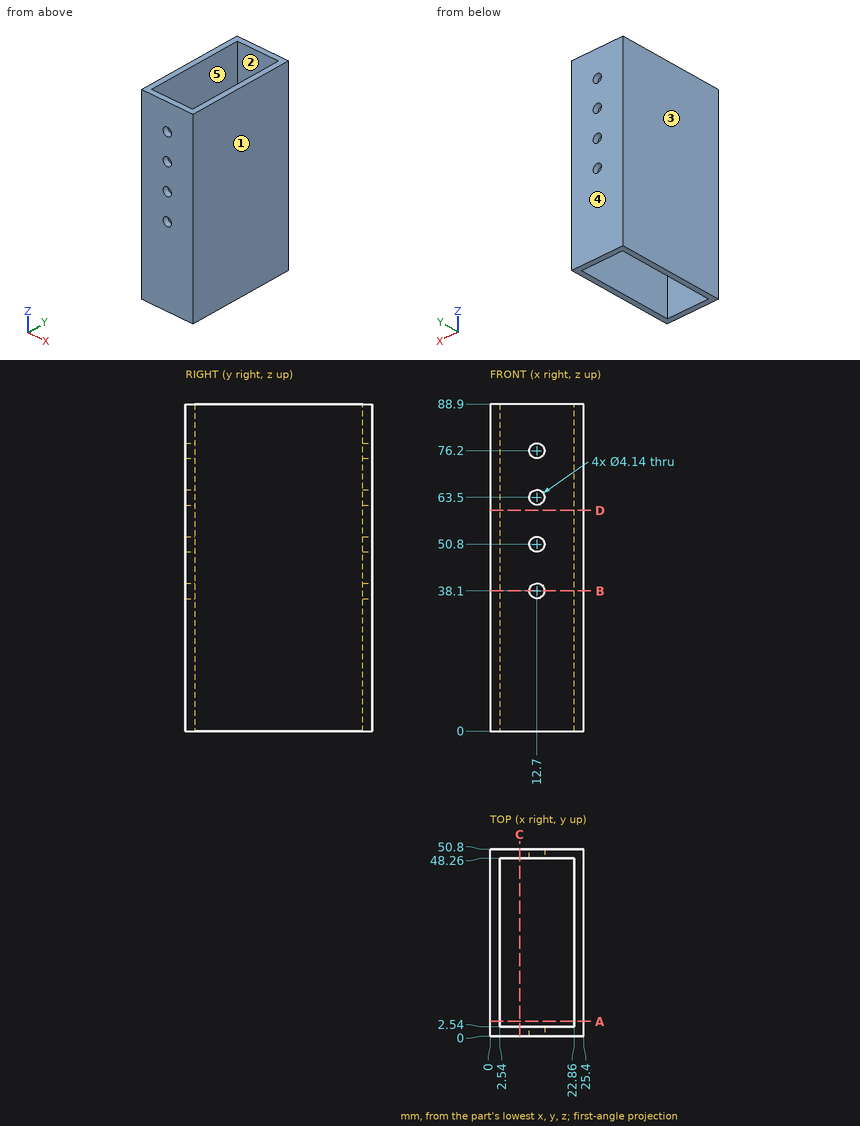
Answer from the drawing. Dimensions are ordinates in mm from the lowest x, y and z of the part. A direction names the side the tool comes from. Round coordinates to 2 decimals unless told otherwise and drop trailing zeros. Loops run counter-clockwise (first coordinate to the right, second up) from the corner with the lowest first, then second, coordinate; pieces in that order, holes last.
Q1. This flat-tipped pin is pushed along its axis until it touches: pin 1 (2.5 mm diameter, centred on x = 12.7, z = 38.1, fed in from +Y). Where does it stop, or does it pass through?
Q2. Determine the mould class of the marked faces 3, 4 and 5 for opening direction Y: released by +Y, released by -Y, zero draft, split by the parting line, or undercut.
Q3. Section D-D on z = 60 is taken. Write down the section's boundary in (x, y), and give its area (3 significant figures).
Q4. Section A-A on y = 4 is taken. Write down the section's boundary in (x, z).
Q5. Section B-B on z = 38.1 is taken. Write down the section's boundary in (x, y).
Q6. Consider probe 1 along Z at (x, y) = (12.7, 0.6); probe 2 along X at (y, z) = (37.5, 16.5); probe 3 along Y at (x, z) = (15.5, 12.5). Determine where each line is inside the solid, lowest interval first.
Q7. Which of the six approach directions +Z, -Z, +X, -X, +Y, -Y give full straight-line access (tool end or side, diameter ignored) to the marked faces 1 and 2?
Q8. Section C-C on x = 8 is taken. Write down the section's boundary in (y, z).
Output:
1. pin 1: passes through
2. face 3: zero draft
2. face 4: released by +Y
2. face 5: undercut
3. outline: (0, 0) - (25.4, 0) - (25.4, 50.8) - (0, 50.8) - close; hole (2.54, 2.54) - (22.86, 2.54) - (22.86, 48.26) - (2.54, 48.26) - close
3. area: 361 mm2
4. outline: (0, 0) - (2.54, 0) - (2.54, 88.9) - (0, 88.9) - close; (22.86, 0) - (25.4, 0) - (25.4, 88.9) - (22.86, 88.9) - close
5. outline: (0, 0) - (10.63, 0) - (10.63, 2.54) - (2.54, 2.54) - (2.54, 48.26) - (10.63, 48.26) - (10.63, 50.8) - (0, 50.8) - close; (14.77, 0) - (25.4, 0) - (25.4, 50.8) - (14.77, 50.8) - (14.77, 48.26) - (22.86, 48.26) - (22.86, 2.54) - (14.77, 2.54) - close
6. probe 1: z = 0 to 36.03, 40.17 to 48.73, 52.87 to 61.43, 65.57 to 74.13, 78.27 to 88.9
6. probe 2: x = 0 to 2.54, 22.86 to 25.4
6. probe 3: y = 0 to 2.54, 48.26 to 50.8
7. face 1: +Z, -Z, +X, +Y, -Y
7. face 2: +Z, -Z
8. outline: (0, 0) - (2.54, 0) - (2.54, 88.9) - (0, 88.9) - close; (48.26, 0) - (50.8, 0) - (50.8, 88.9) - (48.26, 88.9) - close
